The drawing under review shows one solid part. Ordinate dimensions are in mm from its lowest x, y, z. Coordinates: 2 decimals unless noted, no trailing zeros. Loops run counter-clockwise (first coordinate to the right, second up) from the corner with the lowest first, then second, coordinate; pieces in that order, holes last. Notation, with made-up numbers: (42, 77.5) - (84, 77.5) arc R26 cw to (84, 93.5) - close; hole circle Ø8 at (74, -39.75). An arc over 180 degrees is marked (long way). Use one line per item in the form item = value. Start each with the question number.
1. Add section D-D on y = 6. Give the boundary of the cut face in (x, z), and give its area (3 significant figures).
2. For pin 1 Ø14 at (x, z) = (88.5, 5.5) entering from -Y; pin 2 Ø7.5 at (x, z) = (39.5, 53) entering from -Y; pin 3 Ø6.5 at (x, y) = (74, 20.5) entering from +Z, all flat-tipped, find the tip position at first contact; note any pin that passes through.
3. To check wall thickness, follow probe 1 along Y at (x, z) = (42.5, 43.5); probe 2 along Z at (x, y) = (29, 25); probe 3 along Z at (x, y) = (27, 18.5). State the ranges of each line that lie inside material, in increasing order.
4. Add section C-C on y = 22.5. Give the boundary of the cut face in (x, z), and give its area (3 significant figures).
5. Add section A-A on z = 42.5. Give the boundary of the cut face in (x, y).
6. Draft analysis for pull direction Y (two halves, no side actions). For the marked faces 1, 2, 3 and 4, state which applies: +Y half, -Y half, draft (parallel to the pull), parting line (faces both ways), or undercut.
7. Add section B-B on x = 88. Give the boundary of the cut face in (y, z).
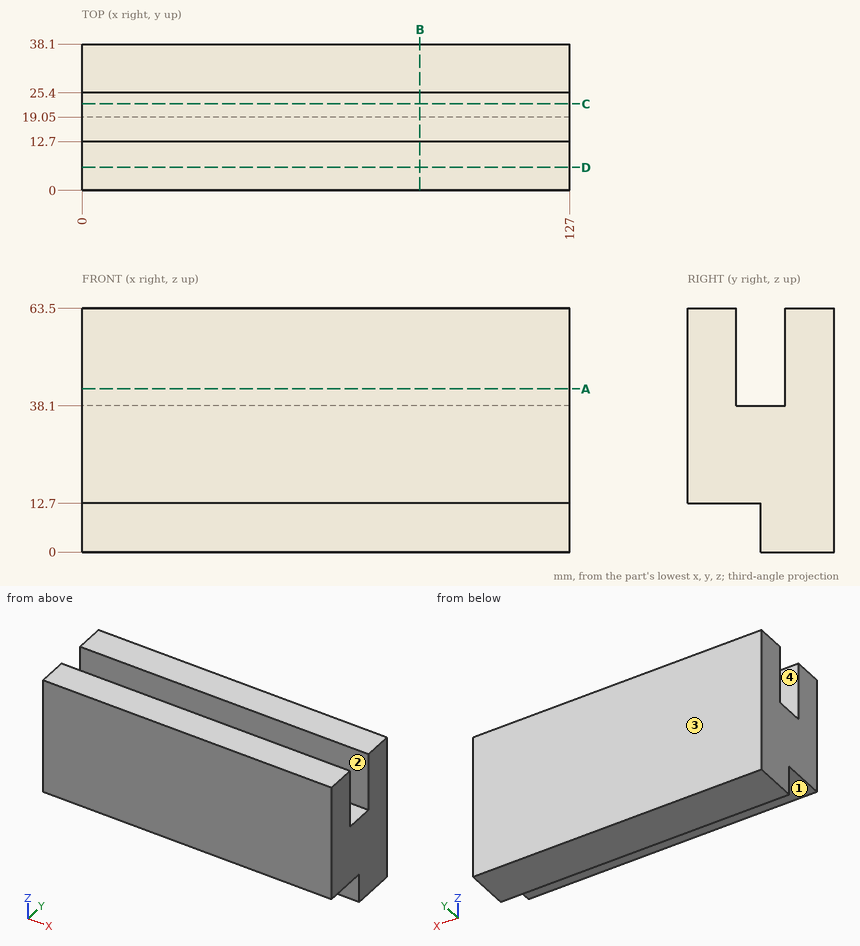
Conclusion:
q1.outline = (0, 12.7) - (127, 12.7) - (127, 63.5) - (0, 63.5) - close
q1.area = 6,450 mm^2
q2.pin_1 = 19.05
q2.pin_2 = 0
q2.pin_3 = 38.1
q3.probe_1 = 0 to 12.7, 25.4 to 38.1
q3.probe_2 = 0 to 38.1
q3.probe_3 = 12.7 to 38.1
q4.outline = (0, 0) - (127, 0) - (127, 38.1) - (0, 38.1) - close
q4.area = 4,840 mm^2
q5.outline = (0, 0) - (127, 0) - (127, 12.7) - (0, 12.7) - close; (0, 25.4) - (127, 25.4) - (127, 38.1) - (0, 38.1) - close
q6.face_1 = draft
q6.face_2 = undercut
q6.face_3 = +Y half
q6.face_4 = undercut
q7.outline = (0, 12.7) - (19.05, 12.7) - (19.05, 0) - (38.1, 0) - (38.1, 63.5) - (25.4, 63.5) - (25.4, 38.1) - (12.7, 38.1) - (12.7, 63.5) - (0, 63.5) - close
